Input: part model. Units: mm. Frame: model coordinates. Coordinates: 2 decimals unless noted, no trailing zeros. Order: outer loops, then holes, each group sorted by start corner. A loop starts at its lowest first (then second) coordinate and runs counter-clockwise, first axis right, second up. Notation, with made-up numbers: (8.5, 43.5) -> (61.5, 43.5) arc R22 cw to (61.5, 55.5) -> close; hole circle Ø1 at (-22, 83). An arc over 180 degrees is marked (long way). One line per question, with ' | ' between items.
```python
from build123d import *

# Parameters (mm, degrees)
SKETCH1_W                  = 330.2
SKETCH1_H                  = 254
SKETCH1_W_2                = 82.55
SKETCH1_H_2                = 184.15
BOSS_EXTRUDE1_DEPTH        = 3.175
FILLET1_R                  = 3.175
F_9_0_196_DIAMETER_HOLE1_D = 4.9784
LPATTERN1_COUNT            = 12
LPATTERN1_PITCH            = 25.4


with BuildPart() as part:
    # Sketch1 → Boss-Extrude1 (new body)
    with BuildSketch(Plane(origin=(0, 0, 0), x_dir=(1, 0, 0), z_dir=(0, 1, 0))):
        Rectangle(SKETCH1_W, SKETCH1_H)
        with Locations((-103.505, 0)):
            Rectangle(SKETCH1_W_2, SKETCH1_H_2, mode=Mode.SUBTRACT)
        Rectangle(SKETCH1_W_2, SKETCH1_H_2, mode=Mode.SUBTRACT)
        with Locations((103.505, 0)):
            Rectangle(SKETCH1_W_2, SKETCH1_H_2, mode=Mode.SUBTRACT)
    extrude(amount=BOSS_EXTRUDE1_DEPTH)

    # Fillet1
    fillet1_edges = [part.edges().sort_by_distance(p)[0] for p in [
        (-144.78, 1.5875, -92.075),
        (-144.78, 1.5875, 92.075),
        (-62.23, 1.5875, 92.075),
        (-62.23, 1.5875, -92.075),
        (-41.275, 1.5875, -92.075),
        (-41.275, 1.5875, 92.075),
        (41.275, 1.5875, 92.075),
        (41.275, 1.5875, -92.075),
        (62.23, 1.5875, -92.075),
        (62.23, 1.5875, 92.075),
        (144.78, 1.5875, 92.075),
        (144.78, 1.5875, -92.075),
        (-165.1, 1.5875, -127),
        (165.1, 1.5875, -127),
        (165.1, 1.5875, 127),
        (-165.1, 1.5875, 127),
    ]]
    fillet(fillet1_edges, radius=FILLET1_R)

    # #9 (0.196) Diameter Hole1 (through all)
    with Locations(Plane(origin=(-139.7, 3.175, 114.3), x_dir=(0, 0, 1), z_dir=(0, 1, 0))):
        with Locations((0, 0), (-228.6, 0)):
            f_9_0_196_diameter_hole1 = Hole(F_9_0_196_DIAMETER_HOLE1_D / 2)

    # LPattern1: #9 (0.196) Diameter Hole1 ×12
    with Locations(*[(i * LPATTERN1_PITCH, 0, 0) for i in range(1, LPATTERN1_COUNT)]):
        add(f_9_0_196_diameter_hole1, mode=Mode.SUBTRACT)


solid = part.part
```
1. Cut plane B-B, the plane x = -98. Return loops of the section in (y, z) (3 decimals), and give its area (3 significant figures).
Recorded:
outline: (0, -127) -> (3.175, -127) -> (3.175, -92.075) -> (0, -92.075) -> close; (0, 92.075) -> (3.175, 92.075) -> (3.175, 127) -> (0, 127) -> close | area: 222 mm^2
2. Cut plane C-C, the plane y = 0.75. State how many separate pieces and enclosed holes the cut face has, and give its area (3 significant figures).
Recorded:
separate pieces: 1 | enclosed holes: 27 | area: 37,800 mm^2
3. Cut plane A-A, the plane z = -25.5. Return loops of the section in (x, y) (3 decimals).
Recorded:
outline: (-165.1, 0) -> (-144.78, 0) -> (-144.78, 3.175) -> (-165.1, 3.175) -> close; (-62.23, 0) -> (-41.275, 0) -> (-41.275, 3.175) -> (-62.23, 3.175) -> close; (41.275, 0) -> (62.23, 0) -> (62.23, 3.175) -> (41.275, 3.175) -> close; (144.78, 0) -> (165.1, 0) -> (165.1, 3.175) -> (144.78, 3.175) -> close
4. Ray query, line 1 (X direction, y = 1.4, z = -14.5) (3 decimals); line 2 (Z direction, x = 139.7, y = 1.3) (3 decimals); line 3 (Z direction, x = 67, y = 1.4) (3 decimals). Return the intervals inside material, ascending. Write a range as [from, to].
Recorded:
line 1: x = [-165.1, -144.78], [-62.23, -41.275], [41.275, 62.23], [144.78, 165.1] | line 2: z = [-127, -116.789], [-111.811, -92.075], [92.075, 111.811], [116.789, 127] | line 3: z = [-127, -92.075], [92.075, 127]
